The listing builds one solid part. Answer for the finished solid, in the listing's coordinates (mm). A direction names the side the tool comes from. Coordinates: 2 decimals unless noted, no trailing zeros. Write each loop counter-clockwise with the first axis right and the second up, starting at its lowest first coordinate (ties: lowest second). Pieces come first, ordered by that corner, then holes. Notation, with made-up numbers: M -25,-27 L -5,-27 A10 cw -5,-13 Z; hole C 10.5,59.25 d2. An arc over 180 degrees is marked long. Answer as a JSON object with one key per item and string values. Group by question number.
from build123d import *

# Parameters (mm, degrees)
SKETCH_3_R                      = 2.8
CUT_EXTRUDE_2_DEPTH             = 4
SKETCH_8_R                      = 1.5
CUT_EXTRUDE_5_DEPTH             = 4
SKETCH_10_W                     = 24
SKETCH_10_H                     = 24
SKETCH_10_W_2                   = 20
SKETCH_10_H_2                   = 20
EXTRUDE_1_DEPTH                 = 15
EXTRUDE_2_DEPTH                 = 15
EXTRUDE_2_DEPTH_BACK            = 12
SKETCH_7_R                      = 5
SKETCH_7_R_2                    = 3.5
SKETCH_7_5_R                    = 3.5
CUT_EXTRUDE_6_DEPTH             = 12.360679775
FILLET_START                    = 6
FILLET_1_DEPTH                  = 15
FILLET_1_2_DEPTH                = 15
CUT_EXTRUDE_7_REACH             = 55.487
CUT_EXTRUDE_7_DIRECTION_2_DEPTH = 54.486637521
SKETCH_15_R                     = 20
EXTRUDE_3_DEPTH                 = 5
CUT_EXTRUDE_START               = -6
CUT_EXTRUDE_9_DEPTH             = 6
SKETCH_17_R                     = 1.5
CUT_EXTRUDE_10_DEPTH            = 8
SKETCH_18_R                     = 2.8
CUT_EXTRUDE_11_DEPTH            = 4


with BuildPart() as part:
    # 草图1 → 旋转1 (revolve)
    with BuildSketch(Plane.XY):
        with BuildLine():
            ThreePointArc((-15.620499352, 6), (-18.061145964, 3.183133409), (-20, 0))
            Line((-20, 0), (0, 0))
            Line((0, 0), (0, 6))
            Line((0, 6), (-15.620499352, 6))
        make_face()
    revolve(axis=Axis((0, 10, 0), (0, -1, 0)))

    # 草图3 → 切除-拉伸2 (cut)
    with BuildSketch(Plane.XZ):
        with Locations(Location((0, 0, 0), (0, 0, 270))):
            Circle(SKETCH_3_R)
    extrude(amount=-CUT_EXTRUDE_2_DEPTH, mode=Mode.SUBTRACT)

    # 草图8 → 切除-拉伸5 (cut)
    with BuildSketch(Plane.XZ.offset(-4)):
        with Locations(Location((0, 0, 0), (0, 0, 270))):
            Circle(SKETCH_8_R)
    extrude(amount=-CUT_EXTRUDE_5_DEPTH, mode=Mode.SUBTRACT)

    # 草图10 → 拉伸-薄壁1 (add)
    with BuildSketch(Plane(origin=(0, 6, 0), x_dir=(1, 0, 0), z_dir=(0, 1, 0))):
        Rectangle(SKETCH_10_W, SKETCH_10_H)
        Rectangle(SKETCH_10_W_2, SKETCH_10_H_2, mode=Mode.SUBTRACT)
    extrude(amount=EXTRUDE_1_DEPTH)

    # 草图7 → 凸台-拉伸2 (add, two sides: drawn at the far end of the back side and taken through both)
    with BuildSketch(Plane(origin=(22.360679775, 0, 0), x_dir=(0, 0, -1), z_dir=(1, 0, 0)).offset(-EXTRUDE_2_DEPTH_BACK)):
        with Locations((0, 13)):
            Circle(SKETCH_7_R)
        with Locations((0, 13)):
            Circle(SKETCH_7_R_2, mode=Mode.SUBTRACT)
    extrude(amount=EXTRUDE_2_DEPTH + EXTRUDE_2_DEPTH_BACK)

    # 草图7<5> → 切除-拉伸6 (cut)
    with BuildSketch(Plane(origin=(22.360679775, 0, 0), x_dir=(0, 0, -1), z_dir=(1, 0, 0))):
        with Locations((0, 13)):
            Circle(SKETCH_7_5_R)
    extrude(amount=-CUT_EXTRUDE_6_DEPTH, mode=Mode.SUBTRACT)

    # 圆角1: read off the stored shape, not the designer's step
    # 圆角1 outline → 圆角1 (cut)
    with BuildSketch(Plane(origin=(0, 0, 0), x_dir=(1, 0, 0), z_dir=(0, 1, 0)).offset(FILLET_START)):
        with BuildLine():
            ThreePointArc((-12, 7), (-10.535533906, 10.535533906), (-7, 12))
            Line((-7, 12), (-12, 12))
            Line((-12, 12), (-12, 7))
        make_face()
        with BuildLine():
            Line((12, 12), (7, 12))
            ThreePointArc((7, 12), (10.535533906, 10.535533906), (12, 7))
            Line((12, 7), (12, 12))
        make_face()
        with BuildLine():
            ThreePointArc((-7, -12), (-10.535533906, -10.535533906), (-12, -7))
            Line((-12, -7), (-12, -12))
            Line((-12, -12), (-7, -12))
        make_face()
        with BuildLine():
            Line((12, -12), (12, -7))
            ThreePointArc((12, -7), (10.535533906, -10.535533906), (7, -12))
            Line((7, -12), (12, -12))
        make_face()
    extrude(amount=FILLET_1_DEPTH, mode=Mode.SUBTRACT)

    # Fillet 1 2 outline → Fillet 1 2 (add)
    with BuildSketch(Plane(origin=(0, 0, 0), x_dir=(1, 0, 0), z_dir=(0, 1, 0)).offset(FILLET_START)):
        with BuildLine():
            Line((10, -10), (10, -5))
            ThreePointArc((10, -5), (8.535533906, -8.535533906), (5, -10))
            Line((5, -10), (10, -10))
        make_face()
        with BuildLine():
            ThreePointArc((5, 10), (8.535533906, 8.535533906), (10, 5))
            Line((10, 5), (10, 10))
            Line((10, 10), (5, 10))
        make_face()
        with BuildLine():
            Line((-10, -10), (-5, -10))
            ThreePointArc((-5, -10), (-8.535533906, -8.535533906), (-10, -5))
            Line((-10, -5), (-10, -10))
        make_face()
        with BuildLine():
            ThreePointArc((-10, 5), (-8.535533906, 8.535533906), (-5, 10))
            Line((-5, 10), (-10, 10))
            Line((-10, 10), (-10, 5))
        make_face()
    extrude(amount=FILLET_1_2_DEPTH)

    # 切除-拉伸7: up to this face of the body (flat: up to its plane)
    cut_extrude_7_end = Plane(part.part.faces().sort_by_distance((0, 13.5, -12))[0])
    # 草图13 → 切除-拉伸7 (cut, up to the picked face)
    with BuildSketch(Plane.XY.offset(12), mode=Mode.PRIVATE) as cut_extrude_7_sk1:
        with BuildLine():
            Line((-4, 17.5), (4, 17.5))
            ThreePointArc((4, 17.5), (5.060660172, 17.060660172), (5.5, 16))
            Line((5.5, 16), (5.5, 12))
            ThreePointArc((5.5, 12), (5.060660172, 10.939339828), (4, 10.5))
            Line((4, 10.5), (-4, 10.5))
            ThreePointArc((-4, 10.5), (-5.060660172, 10.939339828), (-5.5, 12))
            Line((-5.5, 12), (-5.5, 16))
            ThreePointArc((-5.5, 16), (-5.060660172, 17.060660172), (-4, 17.5))
        make_face()
    cut_extrude_7_tool1 = split(extrude(cut_extrude_7_sk1.sketch, amount=-CUT_EXTRUDE_7_REACH, mode=Mode.PRIVATE), bisect_by=cut_extrude_7_end, keep=Keep.BOTH, mode=Mode.PRIVATE)
    add(cut_extrude_7_tool1.solids().sort_by(Axis((0, 14, 12), (0, 0, -1)))[0], mode=Mode.SUBTRACT)

    # 草图13 → 切除-拉伸7 direction 2 (cut)
    with BuildSketch(Plane.XY.offset(12)):
        with BuildLine():
            Line((-4, 17.5), (4, 17.5))
            ThreePointArc((4, 17.5), (5.060660172, 17.060660172), (5.5, 16))
            Line((5.5, 16), (5.5, 12))
            ThreePointArc((5.5, 12), (5.060660172, 10.939339828), (4, 10.5))
            Line((4, 10.5), (-4, 10.5))
            ThreePointArc((-4, 10.5), (-5.060660172, 10.939339828), (-5.5, 12))
            Line((-5.5, 12), (-5.5, 16))
            ThreePointArc((-5.5, 16), (-5.060660172, 17.060660172), (-4, 17.5))
        make_face()
    extrude(amount=CUT_EXTRUDE_7_DIRECTION_2_DEPTH, mode=Mode.SUBTRACT)

    # 草图15 → 凸台-拉伸3 (add)
    with BuildSketch(Plane.XZ):
        with Locations(Location((0, 0, 0), (0, 0, 180))):
            Circle(SKETCH_15_R)
    extrude(amount=EXTRUDE_3_DEPTH)

    # 草图16 → 切除-拉伸9 (cut)
    with BuildSketch(Plane(origin=(0, 6, 0), x_dir=(1, 0, 0), z_dir=(0, 1, 0)).offset(CUT_EXTRUDE_START)):
        with BuildLine():
            Line((-5, -10), (5, -10))
            ThreePointArc((5, -10), (8.535533906, -8.535533906), (10, -5))
            Line((10, -5), (10, 5))
            ThreePointArc((10, 5), (8.535533906, 8.535533906), (5, 10))
            Line((5, 10), (-5, 10))
            ThreePointArc((-5, 10), (-8.535533906, 8.535533906), (-10, 5))
            Line((-10, 5), (-10, -5))
            ThreePointArc((-10, -5), (-8.535533906, -8.535533906), (-5, -10))
        make_face()
    extrude(amount=CUT_EXTRUDE_9_DEPTH, mode=Mode.SUBTRACT)

    # 草图17 → 切除-拉伸10 (cut)
    with BuildSketch(Plane(origin=(0, 0, 0), x_dir=(1, 0, 0), z_dir=(0, 1, 0))):
        with Locations(Location((0, 0, 0), (0, 0, 270))):
            Circle(SKETCH_17_R)
    extrude(amount=-CUT_EXTRUDE_10_DEPTH, mode=Mode.SUBTRACT)

    # 草图18 → 切除-拉伸11 (cut)
    with BuildSketch(Plane.XZ.offset(5)):
        with Locations(Location((0, 0, 0), (0, 0, 270))):
            Circle(SKETCH_18_R)
    extrude(amount=-CUT_EXTRUDE_11_DEPTH, mode=Mode.SUBTRACT)


solid = part.part
Item 1: Consider L1, parallel to Z at x = 5, y = 18.75; L2, parallel to Y at x = 24, z = 0. Determine where each line is inside the solid, lowest interval first. Write a range as from..to.
Item 2: A tool of negligible diameter and unlimited length cuts with its end or side. For faces 1 (the face through (10, 13, -11)), 2 (the face through (-8, 10, 9)), 3 (the face through (0, 6, 13)), 4 (the face through (-12, 13, 0)), 5 (the face through (0, 10.5, -11)), from which of +Z, -Z, +X, -X, +Y, -Y can it reach the whole face along a straight path? Write none if from no direction.
Item 3: For a pull along Z with two mould halves and no side action, classify faces 6 (the face through (0, 10, -12)), 7 (the face through (10, 8, 0)), 8 (the face through (0, 17.5, 11)) as +Z half, -Z half, draft (parallel to the pull), parting line (faces both ways), or undercut.
Item 4: Flat-ended cylindrical pins translate along their axes: pin 1 Ø5 at (x, y) = (1.5, 3.5) entering from -Z; pin 2 Ø1 at (y, z) = (13.5, -11) entering from -X; pin 3 Ø4 at (y, z) = (14, -8) entering from -X; pin 4 Ø15.5 at (y, z) = (16, -1.5) entering from +X. Find the tip coordinate at first contact, or state that the pin passes through.
Item 5: A cutting plane is placed at A-A, the plane z = 0. State how many separate pieces and enclosed holes the cut face has, and give its area (3 significant figures).
Item 6: A cutting plane is placed at D-D, the plane y = 19.25. Write down the section's boundary in (x, z), and give its area (3 significant figures).
Item 7: A cutting plane is placed at C-C, the plane y = 13. Write down the section's boundary in (x, z), and give its area (3 significant figures).
Answer:
{
 "1": {"L1": "-12..-10, 10..12", "L2": "8..9.5, 16.5..18"},
 "2": {"face 1": "-Z, +X, +Y", "face 2": "+Y", "face 3": "none", "face 4": "+Z, -Z, -X, +Y", "face 5": "+Z, -Z"},
 "3": {"face 6": "-Z half", "face 7": "undercut", "face 8": "draft"},
 "4": {"pin 1": "z = -19.42", "pin 2": "x = -10.57", "pin 3": "x = -12", "pin 4": "x = 37.36"},
 "5": {"separate pieces": "3", "enclosed holes": "0", "area": "393 mm2"},
 "6": {"outline": "M -12,-7 A5 ccw -7,-12 L 7,-12 A5 ccw 12,-7 L 12,7 A5 ccw 7,12 L -7,12 A5 ccw -12,7 Z; hole M -10,-5 A5 ccw -5,-10 L 5,-10 A5 ccw 10,-5 L 10,5 A5 ccw 5,10 L -5,10 A5 ccw -10,5 Z", "area": "176 mm2"},
 "7": {"outline": "M -12,-7 A5 ccw -7,-12 L -5.5,-12 L -5.5,-9.97 A5 cw -10,-5 L -10,5 A5 cw -5.5,9.97 L -5.5,12 L -7,12 A5 ccw -12,7 Z; M 5.5,-12 L 7,-12 A5 ccw 12,-7 L 12,-5 L 37.36,-5 L 37.36,-3.5 L 10,-3.5 L 10,-5 A5 cw 5.5,-9.97 Z; M 5.5,9.97 A5 cw 10,5 L 10,3.5 L 37.36,3.5 L 37.36,5 L 12,5 L 12,7 A5 ccw 7,12 L 5.5,12 Z", "area": "194 mm2"}
}
